The listing builds one solid part. Answer for the finished solid, in the listing's coordinates (mm). A direction names the side the tool comes from. Give positions to 0.01 mm unless a question says otherwise; leave off trailing zeros. Loops run counter-clockwise (first coordinate to the right, second up) from the corner with the lowest first, then second, coordinate; pieces in that order, holes last. Notation, with made-up numbers: (55, -0.75) - (72, -0.75) arc R19 cw to (72, 34.25) - close; hole circle Ø9 at (51.25, 76.5). An arc over 180 degrees is marked (long way). Write item = value, one per line. Start each with the question number.
1) The part is cut by section B-B on y = 5.2. Write down the section's boundary in (x, z).
2) Consider probe 1 along Z at (x, y) = (-6, 2.35); probe 2 along X at (y, z) = (5.5, -4.25). Determine where each line is inside the solid, lowest interval first.
3) Which of the six approach directions +Z, -Z, +X, -X, +Y, -Y give full straight-line access (tool end or side, diameter ignored) to faces 4 (the flat face through (-0.1, 6, -12.6)), 5 (the flat face through (-10, 2, 0))?
4) The part is cut by section C-C on x = -5.5. Write down the section's boundary in (y, z).
5) The part is cut by section A-A on y = 1.45. Write down the section's boundary in (x, z).
6) The part is cut by section D-D on z = 5.25. Write down the section's boundary in (x, y).
7) The mould has two halves that part along Z. Classify faces 1 (the flat face through (10, 2, 0)), 2 (the flat face through (0, 3, 13)), 3 (the flat face through (-13, 3, 0)): +Z half, -Z half, draft (parallel to the pull), parting line (faces both ways), or undercut.
8) A flat-ended cylindrical pin translates along its axis: P1, Ø10, axis at x = -3.5, z = 4, coming from the +Y side. Find the tip coordinate at first contact, or state that the pin passes through.
from build123d import *

# Parameters (mm, degrees)
SKETCH1_W           = 20
SKETCH1_H           = 20
BOSS_EXTRUDE1_DEPTH = 4
SKETCH2_W           = 24
SKETCH2_H           = 24
BOSS_EXTRUDE2_DEPTH = 1
SKETCH2_3_W         = 26
SKETCH2_3_H         = 26
SKETCH2_3_W_2       = 24
SKETCH2_3_H_2       = 24
BOSS_EXTRUDE3_DEPTH = 6
FILLET1_R           = 2
FILLET2_R           = 2


with BuildPart() as part:
    # Sketch1 → Boss-Extrude1 (new body)
    with BuildSketch(Plane(origin=(0, 0, 0), x_dir=(1, 0, 0), z_dir=(0, 1, 0))):
        Rectangle(SKETCH1_W, SKETCH1_H)
    extrude(amount=BOSS_EXTRUDE1_DEPTH)

    # Sketch2 → Boss-Extrude2 (add)
    with BuildSketch(Plane(origin=(0, 0, 0), x_dir=(1, 0, 0), z_dir=(0, 1, 0))):
        Rectangle(SKETCH2_W, SKETCH2_H)
    extrude(amount=BOSS_EXTRUDE2_DEPTH)

    # Sketch2<3> → Boss-Extrude3 (add)
    with BuildSketch(Plane(origin=(0, 0, 0), x_dir=(1, 0, 0), z_dir=(0, 1, 0))):
        Rectangle(SKETCH2_3_W, SKETCH2_3_H)
        Rectangle(SKETCH2_3_W_2, SKETCH2_3_H_2, mode=Mode.SUBTRACT)
    extrude(amount=BOSS_EXTRUDE3_DEPTH)

    # Fillet1
    fillet1_edges = [part.edges().sort_by_distance(p)[0] for p in [
        (10, 2.5, 10),
        (-10, 2.5, 10),
        (-10, 2.5, -10),
        (10, 2.5, -10),
    ]]
    fillet(fillet1_edges, radius=FILLET1_R)

    # Fillet2
    fillet2_edges = [part.edges().sort_by_distance(p)[0] for p in [
        (12, 3.5, -12),
        (-12, 3.5, -12),
        (-12, 3.5, 12),
        (12, 3.5, 12),
    ]]
    fillet(fillet2_edges, radius=FILLET2_R)


solid = part.part
Answer below:
q1.outline = (-13, -13) - (13, -13) - (13, 13) - (-13, 13) - close; hole (-12, -10) arc R2 ccw to (-10, -12) - (10, -12) arc R2 ccw to (12, -10) - (12, 10) arc R2 ccw to (10, 12) - (-10, 12) arc R2 ccw to (-12, 10) - close
q2.probe_1 = -13 to -12, -10 to 10, 12 to 13
q2.probe_2 = -13 to -12, 12 to 13
q3.face_4 = +Z, -Z, +X, -X, +Y
q3.face_5 = +Y
q4.outline = (0, -13) - (6, -13) - (6, -12) - (1, -12) - (1, -10) - (4, -10) - (4, 10) - (1, 10) - (1, 12) - (6, 12) - (6, 13) - (0, 13) - close
q5.outline = (-13, -13) - (13, -13) - (13, 13) - (-13, 13) - close; (-10, -8) arc R2 ccw to (-8, -10) - (8, -10) arc R2 ccw to (10, -8) - (10, 8) arc R2 ccw to (8, 10) - (-8, 10) arc R2 ccw to (-10, 8) - close; hole (-12, -10) arc R2 ccw to (-10, -12) - (10, -12) arc R2 ccw to (12, -10) - (12, 10) arc R2 ccw to (10, 12) - (-10, 12) arc R2 ccw to (-12, 10) - close
q6.outline = (-13, 0) - (13, 0) - (13, 6) - (12, 6) - (12, 1) - (10, 1) - (10, 4) - (-10, 4) - (-10, 1) - (-12, 1) - (-12, 6) - (-13, 6) - close
q7.face_1 = undercut
q7.face_2 = +Z half
q7.face_3 = draft
q8.P1 = 4
